```python
from build123d import *

# Parameters (mm, degrees)
BOSS_EXTRUDE1_DEPTH = 2.5
SKETCH16_R          = 2.75
CUT_EXTRUDE2_DEPTH  = 15


with BuildPart() as part:
    # Sketch1 → Boss-Extrude1 (new body)
    with BuildSketch(Plane.XY):
        with BuildLine():
            Line((3.125, -17.5), (3.125, -9.499177596))
            ThreePointArc((3.125, -9.499177596), (7.071067812, -7.071067812), (9.499177596, -3.125))
            Line((9.499177596, -3.125), (17.5, -3.125))
            ThreePointArc((17.5, -3.125), (19.5, 0), (17.5, 3.125))
            Line((17.5, 3.125), (9.499177596, 3.125))
            ThreePointArc((9.499177596, 3.125), (7.071067812, 7.071067812), (3.125, 9.499177596))
            Line((3.125, 9.499177596), (3.125, 17.5))
            ThreePointArc((3.125, 17.5), (0, 19.5), (-3.125, 17.5))
            Line((-3.125, 17.5), (-3.125, 9.499177596))
            ThreePointArc((-3.125, 9.499177596), (-7.071067812, 7.071067812), (-9.499177596, 3.125))
            Line((-9.499177596, 3.125), (-17.5, 3.125))
            ThreePointArc((-17.5, 3.125), (-19.5, 0), (-17.5, -3.125))
            Line((-17.5, -3.125), (-9.499177596, -3.125))
            ThreePointArc((-9.499177596, -3.125), (-7.071067812, -7.071067812), (-3.125, -9.499177596))
            Line((-3.125, -9.499177596), (-3.125, -17.5))
            ThreePointArc((-3.125, -17.5), (0, -19.5), (3.125, -17.5))
        make_face()
        with BuildLine():
            ThreePointArc((-9.868180698, -1.618335477), (-9.86763363, -1.621667831), (-9.867085436, -1.625))
            Line((-9.867085436, -1.625), (-9.878306468, -1.625))
            Line((-9.878306468, -1.625), (-17.120871128, -1.625))
            ThreePointArc((-17.120871128, -1.625), (-18, 0), (-17.120871128, 1.625))
            Line((-17.120871128, 1.625), (-9.878306468, 1.625))
            Line((-9.878306468, 1.625), (-9.867085436, 1.625))
            ThreePointArc((-9.867085436, 1.625), (-9.86763363, 1.621667831), (-9.868180698, 1.618335477))
            ThreePointArc((-9.868180698, 1.618335477), (-8.999177596, 0), (-9.868180698, -1.618335477))
        make_face(mode=Mode.SUBTRACT)
        with BuildLine():
            ThreePointArc((-1.618335477, -9.868180698), (0, -8.999177596), (1.618335477, -9.868180698))
            ThreePointArc((1.618335477, -9.868180698), (1.621667831, -9.86763363), (1.625, -9.867085436))
            Line((1.625, -9.867085436), (1.625, -9.878306468))
            Line((1.625, -9.878306468), (1.625, -17.120871128))
            ThreePointArc((1.625, -17.120871128), (0, -18), (-1.625, -17.120871128))
            Line((-1.625, -17.120871128), (-1.625, -9.878306468))
            Line((-1.625, -9.878306468), (-1.625, -9.867085436))
            ThreePointArc((-1.625, -9.867085436), (-1.621667831, -9.86763363), (-1.618335477, -9.868180698))
        make_face(mode=Mode.SUBTRACT)
        with BuildLine():
            Line((1.625, 9.878306468), (1.625, 9.867085436))
            ThreePointArc((1.625, 9.867085436), (1.621667831, 9.86763363), (1.618335477, 9.868180698))
            ThreePointArc((1.618335477, 9.868180698), (0, 8.999177596), (-1.618335477, 9.868180698))
            ThreePointArc((-1.618335477, 9.868180698), (-1.621667831, 9.86763363), (-1.625, 9.867085436))
            Line((-1.625, 9.867085436), (-1.625, 9.878306468))
            Line((-1.625, 9.878306468), (-1.625, 17.120871128))
            ThreePointArc((-1.625, 17.120871128), (0, 18), (1.625, 17.120871128))
            Line((1.625, 17.120871128), (1.625, 9.878306468))
        make_face(mode=Mode.SUBTRACT)
        with BuildLine():
            ThreePointArc((9.868180698, 1.618335477), (9.86763363, 1.621667831), (9.867085436, 1.625))
            Line((9.867085436, 1.625), (9.878306468, 1.625))
            Line((9.878306468, 1.625), (17.120871128, 1.625))
            ThreePointArc((17.120871128, 1.625), (18, 0), (17.120871128, -1.625))
            Line((17.120871128, -1.625), (9.878306468, -1.625))
            Line((9.878306468, -1.625), (9.867085436, -1.625))
            ThreePointArc((9.867085436, -1.625), (9.86763363, -1.621667831), (9.868180698, -1.618335477))
            ThreePointArc((9.868180698, -1.618335477), (8.999177596, 0), (9.868180698, 1.618335477))
        make_face(mode=Mode.SUBTRACT)
    extrude(amount=BOSS_EXTRUDE1_DEPTH)

    # Loft2: read off the stored shape, not the designer's step
    # Loft2: loft between two sections, ruled curve by curve
    loft2_from = [
        Edge.make_bspline([(3.048060313, 1.127753665, -15), (0.792552983, 7.223874291, -15), (-5.303567643, 4.968366961, -15), (-3.048060313, -1.127753665, -15), (-0.792552983, -7.223874291, -15), (5.303567643, -4.968366961, -15), (3.048060313, 1.127753665, -15)], [0, 0, 0, 0, 0.5, 0.5, 0.5, 1, 1, 1, 1], 3, [1, 0.333333333, 0.333333333, 1, 0.333333333, 0.333333333, 1]),
    ]
    loft2_to = [
        Edge.make_bspline([(4.41488096, 4.063105476, 0), (-3.711329991, 12.892867396, 0), (-12.541091911, 4.766656445, 0), (-4.41488096, -4.063105476, 0), (3.711329991, -12.892867396, 0), (12.541091911, -4.766656445, 0), (4.41488096, 4.063105476, 0)], [0, 0, 0, 0, 0.5, 0.5, 0.5, 1, 1, 1, 1], 3, [1, 0.333333333, 0.333333333, 1, 0.333333333, 0.333333333, 1]),
    ]
    loft2 = Solid(Shell([*[Face.make_surface_from_curves(loft2_from[k], loft2_to[k]) for k in range(1)], Face(Wire(loft2_from)), Face(Wire(loft2_to))]))
    add(loft2)

    # Sketch16 → Cut-Extrude2 (cut)
    with BuildSketch(Plane(origin=(0, 0, -15), x_dir=(-1, 0, 0), z_dir=(0, 0, -1))):
        Circle(SKETCH16_R)
    extrude(amount=-CUT_EXTRUDE2_DEPTH, mode=Mode.SUBTRACT)


solid = part.part
```
Here's how the part is built. I have some questions about the finished solid (model axes, mm). A direction names the side the tool comes from. Coordinates: 2 decimals unless noted, no trailing zeros. Loops run counter-clockwise (first coordinate to the right, second up) from the corner with the lowest first, then second, coordinate; pieces in that order, holes last. Notation, with made-up numbers: (7, 75) -> (12, 75) arc R31 cw to (12, 109) -> close; hole circle Ø9 at (15, -10.75). An arc over 180 degrees is marked (long way). Return JSON: item names as keys, results as strings.
1) If we section it at A-A, the plane y = -12: Write out the boundary of the cut face in (x, z) (3 decimals).
Results below:
{"outline": "(-3.125, 0) -> (-1.625, 0) -> (-1.625, 2.5) -> (-3.125, 2.5) -> close; (1.625, 0) -> (3.125, 0) -> (3.125, 2.5) -> (1.625, 2.5) -> close"}
2) I need wall thicknesses on line 1 (Y direction, x = 0, z = -10.75); line 2 (X direction, y = -0.5, z = -13); line 3 (Z direction, x = -9, y = -3). Which ranges of each line are inside material? Lowest first, please. Write a range as from..to.
Results below:
{"line 1": "-3.95..-2.75, 2.75..3.95", "line 2": "-3.53..-2.7, 2.7..3.53", "line 3": "0..2.5"}
3) If we section it at C-C, the plane x = 0: Count the separate pieces of the cut face and the enclosed holes in it, then the cut area to 3 significant figures.
Results below:
{"separate pieces": "3", "enclosed holes": "0", "area": "107 mm²"}
4) Will these pins go through, and if not, where does the flat tip stop? pin 1 (1 mm diameter, centred on y = -3, z = -6.5, fed in from +X); pin 2 (1.2 mm diameter, centred on x = 14, z = 1, fed in from +Y) (3 decimals); pin 3 (2 mm diameter, centred on x = 14.5, z = 0.5, fed in from -Y) (3 decimals); pin 4 (19.5 mm diameter, centred on x = 5.5, y = 8.5, fed in from -Z).
Results below:
{"pin 1": "x = 4.04", "pin 2": "y = 3.125", "pin 3": "y = -3.125", "pin 4": "z = -15"}
5) For faces 5 (the face through (-13, 3.125, 1)), 6 (the face through (0, 18, 1)), 7 (the face through (0.596, -2.685, -7.605)), which set-ups out of +Z, -Z, +X, -X, +Y, -Y let a thin tool reach every point of the face, with its end or its side?
Results below:
{"face 5": "+Z, -Z, -X, +Y", "face 6": "+Z, -Z", "face 7": "-Z"}
6) Thinking about a two-plate mould opening in X: for faces 1 (the face through (3.125, -14, 1)), 2 (the face through (-9, 0, 1)), 3 (the face through (0, 0, 2.5)), 4 (the face through (-0.1, -19.5, 1.2)), which applies, +X half, -X half, draft (parallel to the pull), parting line (faces both ways), or undercut?
Results below:
{"face 1": "+X half", "face 2": "undercut", "face 3": "draft", "face 4": "parting line"}
